from build123d import *

# Parameters (mm, degrees)
ESQUISSE2_W                  = 15
ESQUISSE2_H                  = 29
ESQUISSE6_R                  = 4.5
ENL_V_MAT_EXTRU_1_DEPTH      = 15
ESQUISSE7_R                  = 2.15
ENL_V_MAT_EXTRU_2_DEPTH      = 66.306967469
R_P_TITION_CIRCULAIRE1_COUNT = 4
ESQUISSE14_W                 = 1.4
ESQUISSE14_H                 = 0.85
ESQUISSE15_R                 = 3
EXTRUSION1_DEPTH             = 75.632432697


with BuildPart() as part:
    # Esquisse2 → Base-Révolution (revolve)
    with BuildSketch(Plane.XY):
        with Locations((-7.5, 14.5)):
            Rectangle(ESQUISSE2_W, ESQUISSE2_H)
    revolve(axis=Axis((10, 0, 0), (-1, 0, 0)))

    # Esquisse4 → Boss.-Révol.1 (revolve)
    with BuildSketch(Plane.XY, mode=Mode.PRIVATE) as boss_r_vol_1_sk:
        Polygon((-15, 3), (-15, 40), (-23, 40), (-23, 35.5), (-27, 35.5), (-51, 25.5), (-51, 3), align=None)
    revolve(boss_r_vol_1_sk.sketch.rotate(Axis((-51, 3, 0), (-1, 0, 0)), 90), axis=Axis((-51, 3, 0), (-1, 0, 0)))

    # Esquisse6 → Enlèv. mat.-Extru.1 (cut)
    with BuildSketch(Plane.ZY.offset(51)):
        with Locations(Location((-16.263455967, 16.263455967, 0), (0, 0, 270))):
            Circle(ESQUISSE6_R)
    enl_v_mat_extru_1 = extrude(amount=-ENL_V_MAT_EXTRU_1_DEPTH, mode=Mode.SUBTRACT)

    # Esquisse7 → Enlèv. mat.-Extru.2 (cut, through all)
    with BuildSketch(Plane.ZY.offset(36)):
        with Locations(Location((-16.263455967, 16.263455967, 0), (0, 0, 270))):
            Circle(ESQUISSE7_R)
    enl_v_mat_extru_2 = extrude(amount=-ENL_V_MAT_EXTRU_2_DEPTH, mode=Mode.SUBTRACT)

    # Répétition circulaire1: Enlèv. mat.-Extru.1, Enlèv. mat.-Extru.2 ×4 about axis
    r_p_tition_circulaire1_axis = Axis((0, 0, 0), (1, 0, 0))
    add([enl_v_mat_extru_1.rotate(r_p_tition_circulaire1_axis, i * 360 / R_P_TITION_CIRCULAIRE1_COUNT) for i in range(1, R_P_TITION_CIRCULAIRE1_COUNT)], mode=Mode.SUBTRACT)
    add([enl_v_mat_extru_2.rotate(r_p_tition_circulaire1_axis, i * 360 / R_P_TITION_CIRCULAIRE1_COUNT) for i in range(1, R_P_TITION_CIRCULAIRE1_COUNT)], mode=Mode.SUBTRACT)

    # Esquisse13 → Enlèvement de matière-Révolution1 (revolve, cut)
    with BuildSketch(Plane.XY):
        Polygon((3, 0), (3, 15), (-18.5, 15), (-18.5, 16), (-51, 16), (-51, 0), align=None)
    revolve(axis=Axis((3, 0, 0), (-1, 0, 0)), mode=Mode.SUBTRACT)

    # Esquisse14 → Enlèvement de matière-Révolution2 (revolve, cut)
    with BuildSketch(Plane.XY):
        with Locations((-49.1, 16.425)):
            Rectangle(ESQUISSE14_W, ESQUISSE14_H)
    revolve(axis=Axis((-44.664297448, 0, 0), (-1, 0, 0)), mode=Mode.SUBTRACT)

    # Esquisse15 → Extrusion1 (cut, through all)
    with BuildSketch(Plane(origin=(0, 0, 0), x_dir=(1, 0, 0), z_dir=(0, 1, 0))):
        with Locations(Location((-12, 0, 0), (0, 0, 180))):
            Circle(ESQUISSE15_R)
    extrude(amount=EXTRUSION1_DEPTH, mode=Mode.SUBTRACT)


solid = part.part
Geometry check sheet. Reference: the model listing, model coordinates, mm. A direction names the side the tool comes from. Give positions to 0.01 mm unless a question says otherwise; leave off trailing zeros. Loops run counter-clockwise (first coordinate to the right, second up) from the corner with the lowest first, then second, coordinate; pieces in that order, holes last.
(1) Set-up check for faces 4 (the flat face through (-36, 17, 14)), 5 (the cylindrical face through (-49.09, -2.194, -16.707)), 6 (the cylindrical face through (-9, 22, 0)): record each of +Z, -Z, +X, -X, +Y, -Y from which the full face is reachable in a straight line by a thin tool's end or side.
From the geometry:
face 4: -X
face 5: none
face 6: +Y
(2) Depth check by flat-ended pin: pin 1 Ø2 at (x, y) = (-21.5, 5) entering from -Z; pin 2 Ø3 at (x, y) = (-41, 28.5) entering from +Z; pin 3 Ø8 at (y, z) = (-16.26, -16.26) entering from -X. Enter the tip coordinate at first touch or a pass-through.
From the geometry:
pin 1: stops at z = -36.99
pin 2: stops at z = 11.94
pin 3: stops at x = -36
(3) Thickness scan on L1, parallel to Y at x = -25, z = 0; L2, parallel to X at y = -19, z = 24.5; L3, parallel to Y at x = -4, z = 0. Record the ranges inside material, lowest first.
From the geometry:
L1: y = -29.5 to -16, 16 to 35.5
L2: x = -23 to -15
L3: y = -29 to -15, 15 to 29
(4) Release check for a two-part mould opening along Z. For faces 1 (the flat face through (-15, 27, 11)), 2 (the cylindrical face through (-18.25, 14.21, -15.62)), 3 (the cylindrical face through (-19.06, 39.12, 8.02)) record: released by +Z, released by -Z, zero draft, split by the parting line, or undercut.
From the geometry:
face 1: zero draft
face 2: undercut
face 3: split by the parting line
(5) Section check A-A on x = -13. Record the cut outline in (y, z).
From the geometry:
outline: (14.73, -2.83) arc R15 cw (long way) to (14.73, 2.83) - (28.86, 2.83) arc R29 ccw (long way) to (28.86, -2.83) - close; hole circle Ø4.3 at (-16.26, -16.26); hole circle Ø4.3 at (-16.26, 16.26); hole circle Ø4.3 at (16.26, -16.26); hole circle Ø4.3 at (16.26, 16.26)
(6) Section check D-D on x = -46. Record the cut outline in (y, z), then the cut area to 3 significant figures.
From the geometry:
outline: (-18.31, -12.26) arc R4.5 cw to (-12.66, -18.95) arc R24.58 ccw to (16.16, -20.76) arc R4.5 cw (long way) to (20.69, -17.07) arc R24.58 ccw to (20.69, 17.07) arc R4.5 cw (long way) to (16.16, 20.76) arc R24.58 ccw to (-12.66, 18.95) arc R4.5 cw to (-18.31, 12.26) arc R24.58 ccw to start; hole circle Ø32 at (0, 0)
area: 924 mm2
(7) Section check C-C on x = -39. Record the cut outline in (y, z).
From the geometry:
outline: (-20.39, -14.46) arc R4.5 cw (long way) to (-15.18, -20.63) arc R27.5 ccw (long way) to (-15.18, 20.63) arc R4.5 cw (long way) to (-20.39, 14.46) arc R27.5 ccw to start; hole circle Ø32 at (0, 0); hole circle Ø9 at (16.26, -16.26); hole circle Ø9 at (16.26, 16.26)
